Geometry check sheet. Reference: drawing and pictorial views, mm from the part's lowest x, y, z. Coordinates: 2 decimals unless noted, no trailing zeros. Loops run counter-clockwise (first coordinate to the right, second up) from the corner with the lowest first, then second, coordinate; pieces in that order, holes last.
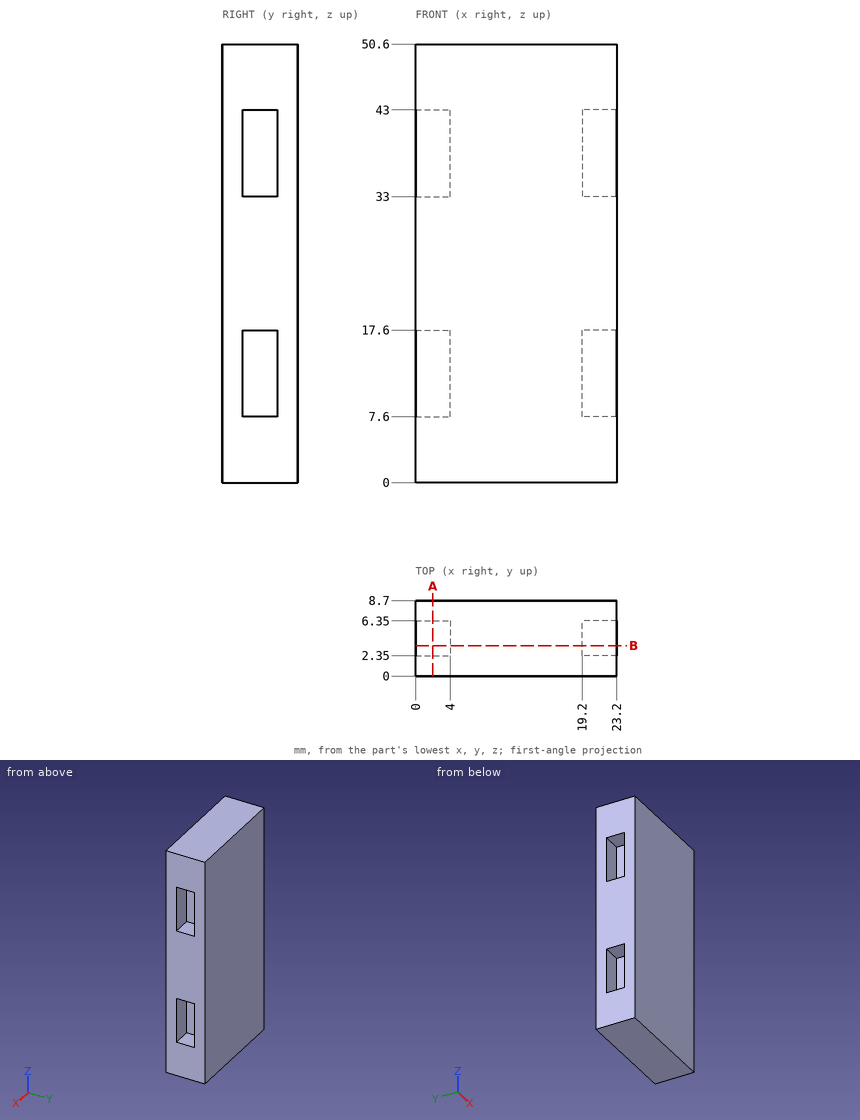
1) Material ranges on probe 1 along Z at (x, y) = (2.25, 4.25); probe 2 along X at (y, z) = (3, 38.5), recorded low to high.
Data:
probe 1: z = 0 to 7.6, 17.6 to 33, 43 to 50.6
probe 2: x = 4 to 19.2
2) Section check B-B on y = 3.5. Record the cut outline in (x, z).
Data:
outline: (0, 0) - (23.2, 0) - (23.2, 7.6) - (19.2, 7.6) - (19.2, 17.6) - (23.2, 17.6) - (23.2, 33) - (19.2, 33) - (19.2, 43) - (23.2, 43) - (23.2, 50.6) - (0, 50.6) - (0, 43) - (4, 43) - (4, 33) - (0, 33) - (0, 17.6) - (4, 17.6) - (4, 7.6) - (0, 7.6) - close
3) Depth check by flat-ended pin: pin 1 (1.5 mm diameter, centred on y = 5, z = 9, fed in from -X); pin 2 (3 mm diameter, centred on x = 3, y = 4.5, fed in from -Z); pin 3 (2 mm diameter, centred on y = 5, z = 37.5, fed in from +X). Enter the tip coordinate at first touch or a pass-through.
Data:
pin 1: stops at x = 4
pin 2: stops at z = 0
pin 3: stops at x = 19.2
4) Section check A-A on x = 2. Record the cut outline in (y, z).
Data:
outline: (0, 0) - (8.7, 0) - (8.7, 50.6) - (0, 50.6) - close; hole (2.35, 7.6) - (6.35, 7.6) - (6.35, 17.6) - (2.35, 17.6) - close; hole (2.35, 33) - (6.35, 33) - (6.35, 43) - (2.35, 43) - close
